Design review of the part built by this model. Coordinates are the model's own, in mm. A direction names the side the tool comes from. Coordinates: 2 decimals unless noted, no trailing zeros. Write each loop counter-clockwise with the first axis right and the second up, starting at its lowest first coordinate (ties: lowest second). Pieces come first, ordered by that corner, then holes.
Q1. Clearance check with flat-ended pins moving along their axes: pin 1 Ø1.8 at (x, z) = (-38.5, 2) entering from +Y; pin 2 Ø1.8 at (x, y) = (-327.5, 50) entering from +Z; pin 3 Ø1.8 at (y, z) = (60.5, 2) entering from -X. State where each tip first meets the part, or that it passes through.
Q2. To check wall thickness, follow probe 1 along Y at (x, z) = (-327, 1.5); probe 2 along Y at (x, z) = (-3, 3.7) (3 decimals); probe 3 along X at (y, z) = (52, 5.35). State the ranges of each line that lie inside material, in increasing order.
Q3. Add section A-A, the plane z = 1.9. Give the number of separate pieces and of enclosed holes in the cut face, plus the area to 3 significant figures.
Q4. The part is to be moulded in two halves that separate along X. For faces 1 (the face through (-324, 14, 3)), 2 (the face through (-56, 29, 3)), 3 (the face through (-167, 0, 3)), say which applies: +X half, -X half, draft (parallel to the pull), parting line (faces both ways), or undercut.
Q5. Add section B-B, the plane x = -205.5. Give the boundary of the cut face in (y, z), plus the area to 3 significant figures.
Q6. Machinability: for faces 4 (the face through (-265, 61, 3)), 5 (the face through (-198, 29, 3)), 6 (the face through (-145, 61, 3)), 7 (the face through (-255.143, 61.9, 4.521)), 8 (the face through (-33, 58, 3)), which of the approach directions +Z, -Z, +X, -X, +Y, -Y give a long, thin tool a straight path to every point of the face, cutting with its end or side? Answer none if there is none.
from build123d import *

# Parameters (mm, degrees)
ESQUISSE1_W             = 330
ESQUISSE1_H             = 64
BOSS_EXTRU_1_DEPTH      = 6
ESQUISSE2_W             = 65
ESQUISSE2_H             = 6
ESQUISSE2_W_2           = 40
ESQUISSE2_W_3           = 6
ESQUISSE2_H_2           = 29
ENL_V_MAT_EXTRU_1_DEPTH = 337.20232004
ESQUISSE3_W             = 3
ESQUISSE3_H             = 20
ESQUISSE3_W_2           = 6
ENL_V_MAT_EXTRU_2_DEPTH = 337.20232004
ESQUISSE4_R             = 1.5
ENL_V_MAT_EXTRU_3_DEPTH = 337.20232004
ESQUISSE5_R             = 2.995
ENL_V_MAT_EXTRU_4_DEPTH = 3


with BuildPart() as part:
    # Esquisse1 → Boss.-Extru.1 (new body)
    with BuildSketch(Plane.XY):
        with Locations((-165, 32)):
            Rectangle(ESQUISSE1_W, ESQUISSE1_H)
    extrude(amount=BOSS_EXTRU_1_DEPTH)

    # Esquisse2 → Enlèv. mat.-Extru.1 (cut, through all)
    with BuildSketch(Plane.XY.offset(6)):
        with Locations((-297.5, 61)):
            Rectangle(ESQUISSE2_W, ESQUISSE2_H)
        with Locations((-205, 61)):
            Rectangle(ESQUISSE2_W_2, ESQUISSE2_H)
        with Locations((-125, 61)):
            Rectangle(ESQUISSE2_W_2, ESQUISSE2_H)
        with Locations((-32.5, 61)):
            Rectangle(ESQUISSE2_W, ESQUISSE2_H)
        with Locations((-327, 14.5)):
            Rectangle(ESQUISSE2_W_3, ESQUISSE2_H_2)
        with Locations((-3, 14.5)):
            Rectangle(ESQUISSE2_W_3, ESQUISSE2_H_2)
    extrude(amount=-ENL_V_MAT_EXTRU_1_DEPTH, mode=Mode.SUBTRACT)

    # Esquisse3 → Enlèv. mat.-Extru.2 (cut, through all)
    with BuildSketch(Plane.XY.offset(6)):
        with Locations((-196.5, 29)):
            Rectangle(ESQUISSE3_W, ESQUISSE3_H)
        with Locations((-53, 29)):
            Rectangle(ESQUISSE3_W_2, ESQUISSE3_H)
    extrude(amount=-ENL_V_MAT_EXTRU_2_DEPTH, mode=Mode.SUBTRACT)

    # Esquisse4 → Enlèv. mat.-Extru.3 (cut, through all)
    with BuildSketch(Plane.XY.offset(6)):
        with Locations((-327, 51)):
            Circle(ESQUISSE4_R)
        with Locations((-327, 36)):
            Circle(ESQUISSE4_R)
        with Locations((-3, 36)):
            Circle(ESQUISSE4_R)
        with Locations((-258, 61)):
            Circle(ESQUISSE4_R)
        with Locations((-232, 61)):
            Circle(ESQUISSE4_R)
        with Locations((-178, 61)):
            Circle(ESQUISSE4_R)
        with Locations((-152, 61)):
            Circle(ESQUISSE4_R)
        with Locations((-98, 61)):
            Circle(ESQUISSE4_R)
        with Locations((-72, 61)):
            Circle(ESQUISSE4_R)
        with Locations((-53, 46)):
            Circle(ESQUISSE4_R)
        with Locations((-53, 12)):
            Circle(ESQUISSE4_R)
        with Locations((-3, 51)):
            Circle(ESQUISSE4_R)
    extrude(amount=-ENL_V_MAT_EXTRU_3_DEPTH, mode=Mode.SUBTRACT)

    # Esquisse5 → Enlèv. mat.-Extru.4 (cut)
    with BuildSketch(Plane.XY.offset(6)):
        with Locations((-3, 36)):
            Circle(ESQUISSE5_R)
        with Locations((-327, 36)):
            Circle(ESQUISSE5_R)
        with Locations((-327, 51)):
            Circle(ESQUISSE5_R)
        with Locations((-258, 61)):
            Circle(ESQUISSE5_R)
        with Locations((-232, 61)):
            Circle(ESQUISSE5_R)
        with Locations((-178, 61)):
            Circle(ESQUISSE5_R)
        with Locations((-152, 61)):
            Circle(ESQUISSE5_R)
        with Locations((-98, 61)):
            Circle(ESQUISSE5_R)
        with Locations((-72, 61)):
            Circle(ESQUISSE5_R)
        with Locations((-53, 46)):
            Circle(ESQUISSE5_R)
        with Locations((-53, 12)):
            Circle(ESQUISSE5_R)
        with Locations((-3, 51)):
            Circle(ESQUISSE5_R)
    extrude(amount=-ENL_V_MAT_EXTRU_4_DEPTH, mode=Mode.SUBTRACT)


solid = part.part
Here are the results:
1. pin 1: stops at y = 58
1. pin 2: stops at z = 3
1. pin 3: stops at x = -265
2. probe 1: y = 29 to 34.5, 37.5 to 49.5, 52.5 to 58
2. probe 2: y = 29 to 33.005, 38.995 to 48.005, 53.995 to 58
2. probe 3: x = -330 to -329.82, -324.18 to -5.82, -0.18 to 0
3. separate pieces: 1
3. enclosed holes: 14
3. area: 19,200 mm2
4. face 1: -X half
4. face 2: undercut
4. face 3: draft
5. outline: (0, 0) - (58, 0) - (58, 6) - (0, 6) - close
5. area: 348 mm2
6. face 4: +Z, -Z, -X, +Y
6. face 5: +Z, -Z
6. face 6: +Z, -Z, +Y
6. face 7: +Z
6. face 8: +Z, -Z, +X, +Y
